from build123d import *

# Parameters (mm, degrees)
BOSS_EXTRUDE1_DEPTH              = 6.35
FILLET1_R                        = 3.175
FILLET2_R                        = 44.45
F_1_4_CLEARANCE_HOLE1_D          = 6.7564
SKETCH4_W                        = 100.0125
SKETCH4_H                        = 155.575
CUT_EXTRUDE1_DEPTH               = 746.989881382
F_27_64_0_42188_DIAMETER_HOLE1_D = 10.715752
FILLET3_R                        = 6.35


with BuildPart() as part:
    # Sketch1 → Boss-Extrude1 (new body)
    with BuildSketch(Plane.XY):
        Polygon((0, 0), (0, 571.5), (379.4125, 571.5), (379.4125, 466.725), (479.425, 466.725), (479.425, 355.6), (428.625, 355.6), (428.625, 403.225), (379.4125, 403.225), (379.4125, 0), align=None)
    extrude(amount=BOSS_EXTRUDE1_DEPTH)

    # Fillet1
    fillet1_edges = [part.edges().sort_by_distance(p)[0] for p in [
        (428.625, 403.225, 3.175),
        (379.4125, 403.225, 3.175),
    ]]
    fillet(fillet1_edges, radius=FILLET1_R)

    # Fillet2
    fillet2_edges = [part.edges().sort_by_distance(p)[0] for p in [
        (379.4125, 466.725, 3.175),
        (479.425, 466.725, 3.175),
    ]]
    fillet(fillet2_edges, radius=FILLET2_R)

    # 1/4 Clearance Hole1 (through all)
    with Locations(Plane(origin=(0, 0, 0), x_dir=(-1, 0, 0), z_dir=(0, 0, -1))):
        with Locations((-118.810746346, 98.250269973), (-302.26, 114.3), (-119.685428778, 90.263601703)):
            Hole(F_1_4_CLEARANCE_HOLE1_D / 2)

    # Sketch4 → Cut-Extrude1 (cut, through all)
    with BuildSketch(Plane(origin=(0, 0, 0), x_dir=(-1, 0, 0), z_dir=(0, 0, -1))):
        with Locations((-429.41875, 433.3875)):
            Rectangle(SKETCH4_W, SKETCH4_H)
    extrude(amount=-CUT_EXTRUDE1_DEPTH, mode=Mode.SUBTRACT)

    # 27/64 (0.42188) Diameter Hole1 (through all)
    with Locations(Plane(origin=(0, 0, 0), x_dir=(-1, 0, 0), z_dir=(0, 0, -1))):
        with Locations((-254, 519.1125), (-52.3875, 381), (-140.462, 210.82)):
            Hole(F_27_64_0_42188_DIAMETER_HOLE1_D / 2)

    # Fillet3
    fillet3_edges = [part.edges().sort_by_distance(p)[0] for p in [
        (0, 0, 3.175),
        (0, 571.5, 3.175),
        (379.4125, 571.5, 3.175),
        (379.4125, 0, 3.175),
    ]]
    fillet(fillet3_edges, radius=FILLET3_R)


solid = part.part
Check sheet for the modelled part. Datum: model origin and axes. Units: mm. Round coordinates to 2 decimals unless told otherwise and drop trailing zeros.
Q1. Scan lines: L1, parallel to Y at x = 51.5, z = 5.25; L2, parallel to Y at x = 144, z = 1. Record each from-to range of solid material in increasing order.
Filled sheet:
L1: y = 0 to 375.72, 386.28 to 571.5
L2: y = 0 to 206.8, 214.84 to 571.5
Q2. Draft check along Y on faces 1 (the face through (192, 290, 6.35)), 2 (the face through (259.11, 520.72, 3.22)), 3 (the face through (139.76, 216.13, 3.22)). Enter one of: pulls with the +Y half, pulls with the -Y half, needs draft (parallel to the pull), parting line crosses it, or undercut.
Filled sheet:
face 1: needs draft
face 2: undercut
face 3: undercut
Q3. Depth check by flat-ended pin: P1, Ø6.5, axis at x = 52.39, y = 381, coming from the -Z side; P2, Ø9, axis at x = 302.26, y = 114.3, coming from the -Z side. Enter the tip coordinate at first touch or a pass-through.
Filled sheet:
P1: passes through
P2: stops at z = 0
